Autodesk Inventor part; units mm, degrees
ref_plane "YZ Plane" through (0, 0, 0) normal (1, 0, 0) x (0, 1, 0)
ref_plane "XZ Plane" through (0, 0, 0) normal (0, 1, 0) x (-1, 0, 0)
ref_plane "XY Plane" through (0, 0, 0) normal (0, 0, 1) x (1, 0, 0)
sketch "Sketch1" plane through (0, 0, 0) normal (0, 1, 0) x (-1, 0, 0)
  line L0 (0, 0) -> (203.2, 0)
  line L1 (203.2, 0) -> (203.2, -142.24)
  line L2 (203.2, -142.24) -> (0, -142.24)
  line L3 (0, -142.24) -> (0, 0)
  dimension "d0" = 203.2
  dimension "d1" = 142.24
extrude "Extrusion1" add sketch "Sketch1" along normal blind 76.2
sketch "Sketch2" plane through (0, 76.2, 0) normal (0, 1, 0) x (1, 0, 0)
  line L0 (-203.2, 0) -> (0, 0)
  line L1 (-203.2, 0) -> (-203.2, 71.12)
  line L2 (-203.2, 142.24) -> (-203.2, 0)
  line L3 (0, 0) -> (0, 142.24)
  line L4 (0, 0) -> (-101.6, 0)
  circle A0 centre (-101.6, 71.12) radius 38.1
  circle A1 centre (-101.6, 71.12) radius 58.42
  circle A2 centre (-101.6, 71.12) radius 31.75
  line L5 (0, 142.24) -> (-203.2, 142.24)
  dimension "d4" = 71.12
  dimension "d6" = 101.6
  dimension "d7" = 76.2
  dimension "d8" = 116.84
  dimension "d9" = 63.5
  dimension "d10" = 71.12
extrude "Extrusion2" cut sketch "Sketch2" against normal blind 6.35 contours A1
sketch "Sketch3" plane through (0, 76.2, 0) normal (0, 1, 0) x (1, 0, 0)
  line L0 (0, 0) -> (-101.6, 0)
  line L1 (-203.2, 0) -> (0, 0)
  line L2 (0, 142.24) -> (-203.2, 142.24)
  line L3 (0, 0) -> (0, 142.24)
  circle A0 centre (-101.5719, 71.12) radius 31.75
  line L4 (-133.3219, 71.12) -> (-129.54, 71.12) construction
  line L5 (-130.036, 73.0239) -> (-126.4684, 73.0239) construction
  line L6 (-133.3219, 71.12) -> (-130.0051, 68.7994)
  line L7 (-130.0051, 68.7994) -> (-132.8994, 65.9574)
  line L8 (-133.3219, 71.1322) -> (-130.005, 73.442)
  line L9 (-130.005, 73.442) -> (-132.8994, 76.2826)
  line L10 (-132.8994, 76.2826) -> (-129.2464, 78.0447)
  line L11 (-129.2464, 78.0447) -> (-131.6634, 81.2473)
  line L12 (-131.6634, 81.2473) -> (-127.8155, 82.305)
  line L13 (-127.8155, 82.305) -> (-129.54, 86.1483)
  line L14 (-129.54, 86.1483) -> (-125.61, 86.4823)
  line L15 (-125.61, 86.4823) -> (-126.7161, 90.5064)
  line L16 (-126.7161, 90.5064) -> (-122.6466, 90.3473)
  line L17 (-122.6466, 90.3473) -> (-123.1432, 94.4168)
  line L18 (-123.1432, 94.4168) -> (-119.1835, 93.5625)
  line L19 (-119.1835, 93.5625) -> (-119.1835, 97.5377)
  line L20 (-119.1835, 97.5377) -> (-115.486, 96.0244)
  line L21 (-115.486, 96.0244) -> (-114.8554, 99.9577)
  line L22 (-114.8554, 99.9577) -> (-111.4463, 97.8843)
  line L23 (-111.4463, 97.8843) -> (-110.657, 101.5424)
  line L24 (-110.657, 101.5424) -> (-107.6807, 98.986)
  line L25 (-107.6807, 98.986) -> (-106.2317, 102.5262)
  line L26 (-106.2317, 102.5262) -> (-103.9961, 99.5445)
  line L27 (-103.9961, 99.5445) -> (-101.6, 102.87)
  line L28 (-130.005, 68.798) -> (-132.8994, 65.9574)
  line L29 (-132.8994, 65.9574) -> (-129.2464, 64.1953)
  line L30 (-129.2464, 64.1953) -> (-131.6634, 60.9927)
  line L31 (-131.6634, 60.9927) -> (-127.8155, 59.935)
  line L32 (-127.8155, 59.935) -> (-129.54, 56.0917)
  line L33 (-129.54, 56.0917) -> (-125.61, 55.7577)
  line L34 (-125.61, 55.7577) -> (-126.7161, 51.7336)
  line L35 (-126.7161, 51.7336) -> (-122.6466, 51.8927)
  line L36 (-122.6466, 51.8927) -> (-123.1432, 47.8232)
  line L37 (-123.1432, 47.8232) -> (-119.1835, 48.6775)
  line L38 (-119.1835, 48.6775) -> (-119.1835, 44.7023)
  line L39 (-119.1835, 44.7023) -> (-115.486, 46.2156)
  line L40 (-115.486, 46.2156) -> (-114.8554, 42.2823)
  line L41 (-114.8554, 42.2823) -> (-111.4463, 44.3557)
  line L42 (-111.4463, 44.3557) -> (-110.657, 40.6976)
  line L43 (-110.657, 40.6976) -> (-107.6807, 43.254)
  line L44 (-107.6807, 43.254) -> (-106.2317, 39.7138)
  line L45 (-106.2317, 39.7138) -> (-103.9961, 42.6955)
  line L46 (-103.9961, 42.6955) -> (-101.6, 39.37)
  line L47 (-73.1943, 68.7985) -> (-70.2466, 65.9445)
  line L48 (-69.8219, 71.1322) -> (-73.1695, 73.4245)
  line L49 (-73.1695, 73.4245) -> (-70.2466, 76.2955)
  line L50 (-70.2466, 76.2955) -> (-73.9311, 78.0745)
  line L51 (-73.9311, 78.0745) -> (-71.4902, 81.2764)
  line L52 (-71.4902, 81.2764) -> (-75.3845, 82.305)
  line L53 (-75.3845, 82.305) -> (-73.6219, 86.1817)
  line L54 (-73.6219, 86.1817) -> (-77.59, 86.4823)
  line L55 (-77.59, 86.4823) -> (-76.4523, 90.5383)
  line L56 (-76.4523, 90.5383) -> (-80.5385, 90.348)
  line L57 (-80.5385, 90.348) -> (-80.038, 94.449)
  line L58 (-80.038, 94.449) -> (-84.0015, 93.5938)
  line L59 (-84.0015, 93.5938) -> (-84.0015, 97.5649)
  line L60 (-84.0015, 97.5649) -> (-87.7172, 96.0441)
  line L61 (-87.7172, 96.0441) -> (-88.3345, 99.9789)
  line L62 (-88.3345, 99.9789) -> (-91.7537, 97.8843)
  line L63 (-91.7537, 97.8843) -> (-92.5392, 101.558)
  line L64 (-92.5392, 101.558) -> (-95.5193, 98.986)
  line L65 (-95.5193, 98.986) -> (-96.9668, 102.5343)
  line L66 (-96.9668, 102.5343) -> (-99.2039, 99.5445)
  line L67 (-99.2039, 99.5445) -> (-101.6, 102.87)
  line L68 (-69.8219, 71.1322) -> (-73.195, 68.798)
  line L69 (-73.195, 68.798) -> (-70.2466, 65.9445)
  line L70 (-70.2466, 65.9445) -> (-73.9536, 64.1953)
  line L71 (-73.9536, 64.1953) -> (-71.4902, 60.9636)
  line L72 (-71.4902, 60.9636) -> (-75.3845, 59.935)
  line L73 (-75.3845, 59.935) -> (-73.6219, 56.0583)
  line L74 (-73.6219, 56.0583) -> (-77.59, 55.7577)
  line L75 (-76.4527, 51.701) -> (-80.5534, 51.8927)
  line L76 (-77.59, 55.7577) -> (-76.4527, 51.701)
  line L77 (-80.5534, 51.8927) -> (-80.0351, 47.7913)
  line L78 (-80.0351, 47.7913) -> (-84.0015, 48.6742)
  line L79 (-84.0015, 48.6742) -> (-84.0015, 44.6736)
  line L80 (-84.0015, 44.6736) -> (-87.714, 46.2156)
  line L81 (-87.714, 46.2156) -> (-88.3345, 42.2611)
  line L82 (-88.3345, 42.2611) -> (-91.7537, 44.3557)
  line L83 (-91.7537, 44.3557) -> (-92.5392, 40.682)
  line L84 (-92.5392, 40.682) -> (-95.5193, 43.254)
  line L85 (-95.5193, 43.254) -> (-96.9683, 39.7055)
  line L86 (-96.9683, 39.7055) -> (-99.2039, 42.6955)
  line L87 (-99.2039, 42.6955) -> (-101.6, 39.37)
  line L88 (-133.3219, 71.1322) -> (-130.005, 68.798)
  line L89 (-130.005, 68.798) -> (-132.8994, 65.9574)
  line L90 (-132.8994, 65.9574) -> (-129.2464, 64.1953)
  line L91 (-129.2464, 64.1953) -> (-131.6634, 60.9927)
  line L92 (-131.6634, 60.9927) -> (-127.8155, 59.935)
  line L93 (-127.8155, 59.935) -> (-129.54, 56.0917)
  line L94 (-126.7161, 51.7336) -> (-122.6466, 51.8927)
  line L95 (-122.6466, 51.8927) -> (-123.1432, 47.8232)
  line L96 (-123.1432, 47.8232) -> (-119.1835, 48.6775)
  line L97 (-119.1835, 48.6775) -> (-119.1835, 44.7023)
  line L98 (-119.1835, 44.7023) -> (-115.486, 46.2156)
  line L99 (-115.486, 46.2156) -> (-114.8554, 42.2823)
  line L100 (-114.8554, 42.2823) -> (-111.4463, 44.3557)
  line L101 (-111.4463, 44.3557) -> (-110.657, 40.6976)
  line L102 (-107.6807, 43.254) -> (-110.657, 40.6976)
  line L103 (-107.6807, 43.254) -> (-106.2317, 39.7138)
  line L104 (-106.2317, 39.7138) -> (-103.9961, 42.6955)
  line L105 (-103.9961, 42.6955) -> (-101.6, 39.37)
  line L106 (-101.6, 39.37) -> (-99.2039, 42.6955)
  line L107 (-99.2039, 42.6955) -> (-96.9683, 39.7055)
  line L108 (-96.9683, 39.7055) -> (-95.5193, 43.254)
  line L109 (-95.5193, 43.254) -> (-92.5392, 40.682)
  line L110 (-92.5392, 40.682) -> (-91.7537, 44.3557)
  line L111 (-91.7537, 44.3557) -> (-88.3345, 42.2611)
  line L112 (-129.2464, 78.0447) -> (-131.6634, 81.2473)
  line L113 (-131.6634, 81.2473) -> (-127.8155, 82.305)
  line L114 (-129.54, 86.1483) -> (-127.8155, 82.305)
  line L115 (-129.54, 86.1483) -> (-125.61, 86.4823)
  line L116 (-125.61, 86.4823) -> (-126.7161, 90.5064)
  line L117 (-71.4902, 81.2764) -> (-73.9311, 78.0745)
  line L118 (-73.9311, 78.0745) -> (-70.2466, 76.2955)
  line L119 (-70.2466, 76.2955) -> (-73.1695, 73.4245)
  line L120 (-73.1695, 73.4245) -> (-69.8219, 71.1322)
  line L121 (-69.8219, 71.1322) -> (-73.1943, 68.7985)
  line L122 (-73.1943, 68.7985) -> (-70.2466, 65.9445)
  line L123 (-70.2466, 65.9445) -> (-73.9536, 64.1953)
  line L124 (-73.9536, 64.1953) -> (-71.4902, 60.9636)
  line L125 (-71.4902, 60.9636) -> (-75.3845, 59.935)
  line L126 (-75.3845, 59.935) -> (-73.6219, 56.0583)
  line L127 (-75.3845, 59.935) -> (-73.6219, 56.0583)
  line L128 (-73.6219, 56.0583) -> (-77.59, 55.7577)
  line L129 (-70.2466, 65.9445) -> (-73.1943, 68.7985)
  line L130 (-73.1943, 68.7985) -> (-69.8219, 71.1322)
  line L131 (-69.8219, 71.1322) -> (-73.1695, 73.4245)
  line L132 (-73.1695, 73.4245) -> (-70.2466, 76.2955)
  line L133 (-70.2466, 76.2955) -> (-73.9311, 78.0745)
  line L134 (-71.4902, 60.9636) -> (-73.9536, 64.1953)
  line L135 (-73.9536, 64.1953) -> (-70.2466, 65.9445)
  line L136 (-70.2466, 65.9445) -> (-73.1943, 68.7985)
  line L137 (-73.1943, 68.7985) -> (-70.2466, 65.9445)
  line L138 (-73.1943, 68.7985) -> (-69.8219, 71.1322)
  line L139 (-69.8219, 71.1322) -> (-73.1695, 73.4245)
  line L140 (-73.1695, 73.4245) -> (-70.2466, 76.2955)
  line L141 (-70.2466, 76.2955) -> (-73.9311, 78.0745)
  line L142 (-69.8219, 71.1322) -> (-73.1695, 73.4245)
  line L143 (-71.4902, 81.2764) -> (-75.3845, 82.305)
  line L144 (-75.3845, 82.305) -> (-73.6219, 86.1817)
  line L145 (-73.6219, 86.1817) -> (-77.59, 86.4823)
  line L146 (-77.59, 86.4823) -> (-76.4523, 90.5383)
  line L147 (-73.6219, 86.1817) -> (-77.59, 86.4823)
  line L148 (-80.5385, 90.348) -> (-76.4523, 90.5383)
  line L149 (-71.4902, 81.2764) -> (-73.9311, 78.0745)
  line L150 (-131.6634, 81.2473) -> (-127.8155, 82.305)
  line L151 (-127.8155, 82.305) -> (-129.54, 86.1483)
  line L152 (-129.54, 86.1483) -> (-127.8155, 82.305)
  line L153 (-129.54, 86.1483) -> (-125.61, 86.4823)
  line L154 (-125.61, 86.4823) -> (-126.7161, 90.5064)
  line L155 (-126.7161, 90.5064) -> (-122.6466, 90.3473)
  line L156 (-122.6466, 90.3473) -> (-123.1432, 94.4168)
  line L157 (-123.1432, 94.4168) -> (-122.6466, 90.3473)
  line L158 (-123.1432, 94.4168) -> (-119.1835, 93.5625)
  line L159 (-119.1835, 93.5625) -> (-119.1835, 97.5377)
  line L160 (-119.1835, 97.5377) -> (-115.486, 96.0244)
  line L161 (-115.486, 96.0244) -> (-114.8554, 99.9577)
  line L162 (-114.8554, 99.9577) -> (-111.4463, 97.8843)
  dimension "d13" = 63.5
  dimension "d27" = 69.832
  dimension "d28" = 70.214
  dimension "d29" = 79.316
  dimension "d30" = 78.709
  dimension "d31" = 77.824
extrude "Extrusion3" cut sketch "Sketch3" against normal blind 6.35 contours L68 L47 L70 L71 L72 L73 L74 L76 L75 L77 L78 L79 L80 L81 L82 L83 L84 L85 L86 L87 L46 L45 L44 L43 L42 L41 L40 L39 L38 L37 L36 L35 L34 L33 L32 L31 L30 L29 L7 L88 L8 L9 L10 L11 L12 L13 L14 L15 L16 L17 L18 L19 L20 L21 L22 L23 L24 L25 L26 L27 L67 L66 L65 L64 L63 L62 L61 L60 L59 L58 L57 L56 L55 L54 L53 L52 L51 L50 L49 L48 | A0 L88 L6
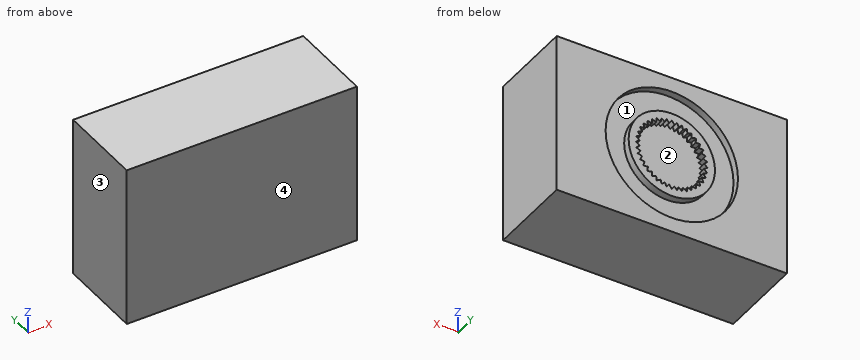
Geometry check sheet. Reference: the model listing, model coordinates, mm. Face numbers are marked on the shaded views. Round coordinates to 2 decimals unless told otherwise and drop trailing zeros. Write each loop counter-clockwise with the first axis right and the second up, starting at its lowest first coordinate (ties: lowest second). Pieces come first, ordered by that corner, then holes.
Item 1: Mould release check, pull along X, two halves, no side actions. Record for the marked faces 1, 2, 3 and 4: +X half, -X half, draft (parallel to the pull), parting line (faces both ways), or undercut.
Determined:
face 1: undercut
face 2: undercut
face 3: -X half
face 4: draft
Item 2: Material ranges on line 1 along X through (y, z) = (71, -71.12); line 2 along Z through (x, y) = (-101.6, 71.5); line 3 along X through (y, z) = (71, -71), recorded low to high.
Determined:
line 1: x = -203.2 to -160.02, -139.7 to -133.32, -69.84 to -63.5, -43.18 to 0
line 2: z = -142.24 to -129.54, -109.22 to -102.87, -39.37 to -33.02, -12.7 to 0
line 3: x = -203.2 to -160.02, -139.7 to -133.15, -70.01 to -63.5, -43.18 to 0
Item 3: Section check A-A (z = -36). Record the boundary of the cut face in (x, y).
Determined:
outline: (-203.2, 0) - (0, 0) - (0, 76.2) - (-54.92, 76.2) - (-54.92, 69.85) - (-86.83, 69.85) - (-86.83, 76.2) - (-116.37, 76.2) - (-116.37, 69.85) - (-148.28, 69.85) - (-148.28, 76.2) - (-203.2, 76.2) - close
